Design review of the part built by this model. Coordinates are the model's own, in mm. A direction names the side the tool comes from. Coordinates: 2 decimals unless noted, no trailing zeros. Write each loop counter-clockwise with the first axis right and the second up, starting at its lowest first coordinate (ties: lowest second). Pieces come first, ordered by that corner, then holes. Notation, with made-up numbers: (47.25, 24.5) - (61.25, 24.5) arc R18 cw to (61.25, 33.5) - close; hole circle Ø2 at (-29, 51). An arc over 180 degrees is marked (long way). One line per item, written item: value.
Solid Edge part; units mm, degrees
sketch "Sketch1" plane through (0, 0, 0) normal (0, 0, 1) x (1, 0, 0)
  line L0 (0, 19.5) -> (0, 6.5)
  line L1 (13, 6.5) -> (13, 19.5)
  arc A0 (13, 6.5) -> (0, 6.5) centre (6.5, 6.5) cw
  arc A1 (0, 19.5) -> (13, 19.5) centre (6.5, 19.5) cw
extrude "Protrusion1" add sketch "Sketch1" along normal blind 6.5
sketch "Sketch2" plane through (6.5, 0, 0) normal (1, 0, 0) x (0, 1, 0)
  line L0 (3.5, 0) -> (3.5, 1)
  line L1 (3.5, 1) -> (2.6811, 3.25)
  line L2 (3.5, 5.5) -> (2.6811, 3.25)
  line L3 (3.5, 6.5) -> (3.5, 5.5)
  line L4 (6.5, 6.5) -> (3.5, 6.5)
  line L5 (6.5, 6.5) -> (6.5, 0)
  line L6 (3.5, 0) -> (6.5, 0)
revolve "RevolvedCutout1" cut sketch "Sketch2" angle 360 about axis through (6.5, 6.5, 6.5) along (0, 0, -1)
chamfer "Chaflán_2" distance 0.75 angle 45 2 edges at (9.5, 6.5, 6.5) (9.5, 6.5, 0)
pattern_linear "Pattern1" count 2 spacing 13 along (0, 1, 0) of "RevolvedCutout1", "Chaflán_2"
chamfer "Chaflán_37" distance 1.5 angle 45 8 edges at (0, 13, 0) (6.5, 26, 0) (13, 13, 0) (6.5, 0, 0) (0, 13, 6.5) (6.5, 26, 6.5) (13, 13, 6.5) (6.5, 0, 6.5)
1. Consider section B-B, the plane z = 2.75. Write out the cut boundary in (x, y).
Answer block:
outline: (0, 6.5) arc R6.5 ccw to (13, 6.5) - (13, 19.5) arc R6.5 ccw to (0, 19.5) - close; hole circle Ø7.27 at (6.5, 6.5); hole circle Ø7.27 at (6.5, 19.5)
2. Consider section A-A, the plane x = 6.5. Give the number of separate pieces and of enclosed holes in the cut face, then the cut area to 3 significant figures.
Answer block:
separate pieces: 3
enclosed holes: 0
area: 76.9 mm^2
3. Wall thickness on line 1 along Y through (x, z) = (9, 3); line 2 along Y through (x, z) = (6.5, 0.85); line 3 along X through (y, z) = (5.75, 1): over which ranges is each line inside the solid? List them lowest first.
Answer block:
line 1: y = 0.5 to 3.73, 9.27 to 16.73, 22.27 to 25.5
line 2: y = 0.65 to 3.5, 9.5 to 16.5, 22.5 to 25.35
line 3: x = 0.55 to 3.6, 9.4 to 12.45
4. Consider section D-D, the plane z = 4. Write out the cut boundary in (x, y), then the cut area to 3 significant figures.
Answer block:
outline: (0, 6.5) arc R6.5 ccw to (13, 6.5) - (13, 19.5) arc R6.5 ccw to (0, 19.5) - close; hole circle Ø7.09 at (6.5, 6.5); hole circle Ø7.09 at (6.5, 19.5)
area: 223 mm^2
5. Insertion check: pin 1 Ø7 at (x, y) = (6.5, 6.5) entering from -Z; pin 2 Ø2 at (x, z) = (10.5, 1.5) entering from -Y; pin 3 Ø1.5 at (x, z) = (11.5, 3.5) entering from +Y. Each pin has a flat end and moves straight along its axis. Give the tip position at first contact, or say it passes through.
Answer block:
pin 1: stops at z = 0.25
pin 2: stops at y = 0.73
pin 3: stops at y = 24.42
6. For faces 4 (the face through (8.357, 8.921, 5.359)), 5 (the face through (6, 13, 6.5)), list the 3-axis set-ups (+Z, -Z, +X, -X, +Y, -Y) from which the entire face can be reached by the end or side of a thin tool; tool diameter is ignored.
Answer block:
face 4: none
face 5: +Z, +X, -X, +Y, -Y
7. Mouldability with a two-part tool opening along Z and no side actions: class faces 1 (the face through (6.6, 1.2, 6.2)), 2 (the face through (4.643, 8.921, 1.141)), 3 (the face through (6.6, 0, 3.2)) as released by +Z, released by -Z, zero draft, split by the parting line, or undercut.
Answer block:
face 1: released by +Z
face 2: undercut
face 3: zero draft
